```python
from build123d import *

# Parameters (mm, degrees)
SKETCH1_R           = 29
BOSS_EXTRUDE1_DEPTH = 10
SKETCH2_W           = 24
SKETCH2_H           = 24
SKETCH2_R           = 10
BOSS_EXTRUDE2_DEPTH = 16
SKETCH3_R           = 3
CUT_EXTRUDE1_DEPTH  = 42
FILLET1_R           = 5
FILLET2_R           = 2
SKETCH4_R           = 1


with BuildPart() as part:
    # Sketch1 → Boss-Extrude1 (new body)
    with BuildSketch(Plane(origin=(0, 0, 0), x_dir=(1, 0, 0), z_dir=(0, 1, 0))):
        Circle(SKETCH1_R)
    extrude(amount=BOSS_EXTRUDE1_DEPTH)

    # Sketch2 → Boss-Extrude2 (add)
    with BuildSketch(Plane.XZ):
        Rectangle(SKETCH2_W, SKETCH2_H)
        Circle(SKETCH2_R, mode=Mode.SUBTRACT)
    extrude(amount=BOSS_EXTRUDE2_DEPTH)

    # Sketch3 → Cut-Extrude1 (cut, through all)
    with BuildSketch(Plane(origin=(12, 0, 0), x_dir=(0, 0, -1), z_dir=(1, 0, 0))):
        with Locations((0, -8)):
            Circle(SKETCH3_R)
    extrude(amount=-CUT_EXTRUDE1_DEPTH, mode=Mode.SUBTRACT)

    # Fillet1
    fillet1_edges = [part.edges().sort_by_distance(p)[0] for p in [
        (12, -8, -12),
        (12, -8, 12),
        (-12, -8, 12),
        (-12, -8, -12),
    ]]
    fillet(fillet1_edges, radius=FILLET1_R)

    # Fillet2
    fillet2_edges = [part.edges().sort_by_distance(p)[0] for p in [
        (0, 0, -12),
        (-12, 0, 0),
        (12, 0, 0),
        (0, 0, 12),
        (-10.535533906, 0, -10.535533906),
        (10.535533906, 0, -10.535533906),
        (10.535533906, 0, 10.535533906),
        (-10.535533906, 0, 10.535533906),
    ]]
    fillet(fillet2_edges, radius=FILLET2_R)

    # Sketch4 → Cut-Revolve1 (revolve, cut)
    with BuildSketch(Plane.XY):
        with Locations((-29, 8)):
            Circle(SKETCH4_R)
    revolve(axis=Axis((0, 0, 0), (0, 1, 0)), mode=Mode.SUBTRACT)


solid = part.part
```
Input: part model. Units: mm. Frame: model coordinates. A direction names the side the tool comes from. Coordinates: 2 decimals unless noted, no trailing zeros. Loops run counter-clockwise (first coordinate to the right, second up) from the corner with the lowest first, then second, coordinate; pieces in that order, holes last. Notation, with made-up numbers: M 43.25,-4 L 93.25,-4 A30 ccw 93.25,18 Z; hole C 15,85 d9. An arc over 180 degrees is marked long. One line per item, written item: value.
(1) Section D-D (y = -3.75). Output: boundary loops of the cut face in (x, z), and give its area (3 significant figures).
Filled in:
outline: M -12,-7 A5 ccw -7,-12 L 7,-12 A5 ccw 12,-7 L 12,7 A5 ccw 7,12 L -7,12 A5 ccw -12,7 Z; hole C 0,0 d20
area: 240 mm^2
(2) Section C-C (x = 0). Output: boundary loops of the cut face in (y, z).
Filled in:
outline: M -16,-12 L -2,-12 A2 cw 0,-14 L 0,-29 L 7,-29 A1 cw 9,-29 L 10,-29 L 10,29 L 9,29 A1 cw 7,29 L 0,29 L 0,14 A2 cw -2,12 L -16,12 L -16,10 L 0,10 L 0,-10 L -16,-10 Z
(3) Section B-B (z = 0). Output: boundary loops of the cut face in (x, y), and give its area (3 significant figures).
Filled in:
outline: M -29,0 L -14,0 A2 cw -12,-2 L -12,-5 L -10,-5 L -10,0 L 10,0 L 10,-5 L 12,-5 L 12,-2 A2 cw 14,0 L 29,0 L 29,7 A1 cw 29,9 L 29,10 L -29,10 L -29,9 A1 cw -29,7 Z; M -12,-16 L -10,-16 L -10,-11 L -12,-11 Z; M 10,-16 L 12,-16 L 12,-11 L 10,-11 Z
area: 619 mm^2
(4) Reachability of faces 1 (the cylindrical face through (11, -9, -10)), 2 (the cylindrical face through (-11, -9, -10)), 3 (the flat face through (12, -12, 0)), 4 (the cylindrical face through (10, -9, 11)) from +Z, -Z, +X, -X, +Y, -Y: full face, straight path, thin tool, end or side. Return the list, or none.
Filled in:
face 1: -Z, +X, -Y
face 2: -Z, -X, -Y
face 3: +Z, -Z, +X, -Y
face 4: +Z, +X, -Y
(5) Line query: line 1 along Y through (x, z) = (10.45, 0); line 2 along X through (y, z) = (-3.5, 0); line 3 along Z through (x, y) = (10.1, -8). Output: solid intervals per line, ascending. Write a range as from..to.
Filled in:
line 1: -16..-11, -5..10
line 2: -12..-10, 10..12
line 3: -10.92..-3, 3..10.92
(6) Pin query (flat end, axial travel): pin 1 (1.5 mm diameter, centred on x = -3, y = -11, fed in from -Z); pin 2 (15.5 mm diameter, centred on x = 2.5, y = -9.5, fed in from +Z); pin 3 (8 mm diameter, centred on y = -8, z = 0, fed in from +X); pin 4 (8 mm diameter, centred on y = -11, z = -17.5, fed in from +X). Return the tip coordinate at first contact, or that it passes through.
Filled in:
pin 1: z = -12
pin 2: z = 12.02
pin 3: x = 12
pin 4: through
(7) Section A-A (y = -8). Output: boundary loops of the cut face in (x, z).
Filled in:
outline: M -12,-7 A5 ccw -7,-12 L 7,-12 A5 ccw 12,-7 L 12,-3 L 9.54,-3 A10 cw -9.54,-3 L -12,-3 Z; M -12,3 L -9.54,3 A10 cw 9.54,3 L 12,3 L 12,7 A5 ccw 7,12 L -7,12 A5 ccw -12,7 Z
(8) Pull-direction query (X, two-part tool) for faces 5 (the flat face through (0, -9, 12)), 6 (the cylindrical face through (9.237, -7.888, -3.83)), 7 (the cylindrical face through (-11, -9, 10)), 8 (the flat face through (0, 0, 0)); classes: +X half, -X half, draft (parallel to the pull), parting line (faces both ways), or undercut.
Filled in:
face 5: draft
face 6: undercut
face 7: -X half
face 8: undercut
